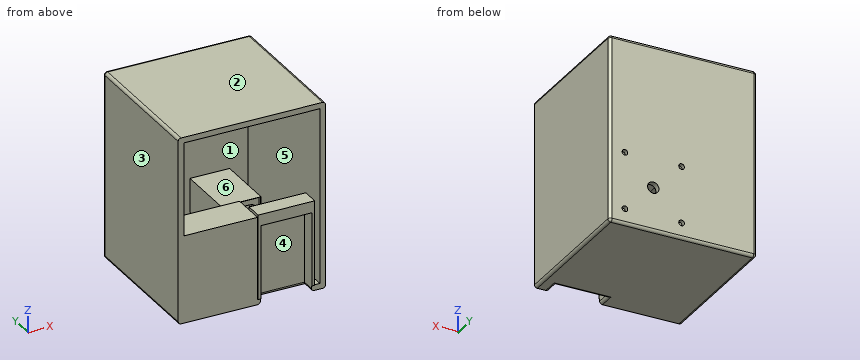
Autodesk Inventor part; units mm, degrees
ref_plane "YZ Plane" through (0, 0, 0) normal (1, 0, 0) x (0, 1, 0)
ref_plane "XZ Plane" through (0, 0, 0) normal (0, 1, 0) x (-1, 0, 0)
ref_plane "XY Plane" through (0, 0, 0) normal (0, 0, 1) x (1, 0, 0)
sketch "Sketch1" plane through (0, 0, 0) normal (0, 1, 0) x (-1, 0, 0)
  line L0 (130, 165) -> (-130, 165)
  line L1 (-130, 165) -> (-130, -165)
  line L2 (-130, -165) -> (130, -165)
  line L3 (130, -165) -> (130, 165)
  point P0 (0, 0)
  point P1 (0, -165)
  point P2 (-130, 0)
  dimension "d0" = 260
  dimension "d1" = 330
extrude "Extrusion1" add sketch "Sketch1" along normal blind 250
sketch "Sketch2" plane through (0, 0, 0) normal (0, -1, 0) x (1, 0, 0)
  line L0 (-120, 155) -> (120, 155)
  line L1 (120, 155) -> (120, -155)
  line L2 (120, -155) -> (-120, -155)
  line L3 (-120, -155) -> (-120, 155)
  line L4 (-130, 165) -> (130, 165)
  line L5 (130, 165) -> (130, -165)
  point P0 (0, 0)
  point P1 (0, 155)
  point P2 (-120, 0)
  dimension "d4" = 10
  dimension "d5" = 10
extrude "Extrusion2" cut sketch "Sketch2" against normal blind 240
fillet "Fillet1" radius 5 8 edges at (0, 250, 165) (-130, 250, 0) (130, 250, 0) (0, 250, -165) (130, 125, -165) (130, 125, 165) (-130, 125, 165) (-130, 125, -165)
sketch "Sketch3" plane through (0, 250, 0) normal (0, 1, 0) x (1, 0, 0)
  circle A0 centre (2.5, 37.5) radius 5
  circle A1 centre (2.5, 137.5) radius 5
  circle A2 centre (102.5, 37.5) radius 5
  circle A3 centre (102.5, 137.5) radius 5
  line L0 (125, 160) -> (125, -160)
  line L1 (-125, 160) -> (125, 160)
  circle A4 centre (52.5, 87.5) radius 10
  point P0 (0, 0)
  dimension "d9" = 10
  dimension "d10" = 10
  dimension "d11" = 10
  dimension "d12" = 10
  dimension "d13" = 100
  dimension "d14" = 100
  dimension "d15" = 22.5
  dimension "d16" = 22.5
  dimension "d19" = 20
  dimension "d20" = 50
  dimension "d21" = 50
extrude "Extrusion3" cut sketch "Sketch3" against normal blind 8
sketch "Sketch4" plane through (52.5, 242, -87.5) normal (0, 1, 0) x (1, 0, 0)
  circle A0 centre (0, 0) radius 10
  circle A1 centre (0, 0) radius 15
  point P0 (-52.5, -87.5)
extrude "Extrusion4" cut sketch "Sketch4" against normal up to next contours A0
sketch "Sketch5" plane through (0, 240, 0) normal (0, -1, 0) x (1, 0, 0)
  line L0 (87.5, -117.5) -> (17.5, -117.5)
  line L1 (17.5, -117.5) -> (17.5, -57.5)
  line L2 (17.5, -57.5) -> (87.5, -57.5)
  line L3 (87.5, -57.5) -> (87.5, -117.5)
  line L4 (120, -155) -> (-120, -155)
  circle A0 centre (52.5, -87.5) radius 15
  circle A1 centre (52.5, -87.5) radius 10
  point P0 (0, 0)
  point P1 (17.5, -87.5)
  point P2 (52.5, -57.5)
  point P3 (52.5, -117.5)
  dimension "d24" = 70
  dimension "d25" = 60
  dimension "d52" = 70
extrude "Extrusion5" add sketch "Sketch5" along normal blind 150 contours L0 L1 L2 L3
sketch "Sketch7" plane through (0, 90, 0) normal (0, -1, 0) x (1, 0, 0)
  line L0 (85, -105) -> (20, -105)
  line L1 (20, -105) -> (20, -70)
  line L2 (20, -70) -> (85, -70)
  line L3 (85, -70) -> (85, -105)
  line L4 (17.5, -117.5) -> (87.5, -117.5)
  line L5 (17.5, -57.5) -> (17.5, -117.5)
  point P0 (0, 0)
  point P1 (52.5, -105)
  point P2 (52.5, -117.5)
  point P3 (52.5, -117.5)
  point P4 (17.5, -87.5)
  point P5 (20, -87.5)
  point P6 (100, -102.5)
  dimension "d28" = 65
  dimension "d29" = 35
extrude "Extrusion6" cut sketch "Sketch7" against normal blind 150
sketch "Sketch8" plane through (0, 240, 0) normal (0, -1, 0) x (1, 0, 0)
  point P0 (0, 0)
sketch "Sketch9" plane through (0, 240, 0) normal (0, -1, 0) x (1, 0, 0)
  circle A0 centre (67, -87.5) radius 2.5
  circle A1 centre (38, -87.5) radius 2.5
  circle A2 centre (52.5, -87.5) radius 10
  circle A3 centre (52.5, -87.5) radius 10
  point P0 (0, 0)
  dimension "d32" = 5
  dimension "d33" = 5
  dimension "d43" = 14.5
  dimension "d44" = 14.5
extrude "Extrusion7" add sketch "Sketch9" along normal up to surface (150 mm away) contours A0 | A1
fillet "Fillet2" radius 15 4 edges at (20, 165, -70) (20, 165, -105) (85, 165, -70) (85, 165, -105)
sketch "Sketch10" plane through (0, 90, 0) normal (0, -1, 0) x (1, 0, 0)
  point P0 (0, 0)
sketch "Sketch11" plane through (0, 90, 0) normal (0, -1, 0) x (1, 0, 0)
  line L0 (18.5, -58.5) -> (86.5, -58.5)
  line L1 (86.5, -58.5) -> (86.5, -116.5)
  line L2 (86.5, -116.5) -> (18.5, -116.5)
  line L3 (18.5, -116.5) -> (18.5, -58.5)
  line L4 (17.5, -57.5) -> (17.5, -117.5)
  line L5 (87.5, -117.5) -> (87.5, -57.5)
  line L6 (87.5, -57.5) -> (17.5, -57.5)
  line L7 (17.5, -117.5) -> (87.5, -117.5)
  point P0 (0, 0)
  point P1 (100, -42.5)
  point P2 (100, -102.5)
  dimension "d46" = 1
  dimension "d47" = 1
  dimension "d48" = 1
  dimension "d49" = 1
extrude "Extrusion8" add sketch "Sketch11" along normal blind 5
sketch "Sketch12" plane through (-120, 0, 155) normal (1, 0, 0) x (0, 0, -1)
  line L0 (315, 0) -> (165, 0)
  line L1 (165, 0) -> (165, 60)
  line L2 (165, 60) -> (315, 60)
  line L3 (315, 60) -> (315, 0)
  line L4 (315, 245) -> (315, 0)
  point P0 (155, 0)
  dimension "d53" = 150
  dimension "d54" = 60
  dimension "d57" = 0
extrude "Extrusion9" add sketch "Sketch12" along normal blind 130
sketch "Sketch15" plane through (0, 85, 0) normal (0, -1, 0) x (1, 0, 0)
  line L0 (97.9773, -47.1324) -> (13.5699, -47.1324)
  line L1 (13.5699, -47.1324) -> (13.5699, -120.1648)
  line L2 (13.5699, -120.1648) -> (97.9773, -120.1648)
  line L3 (97.9773, -120.1648) -> (97.9773, -47.1324)
  point P0 (0, 0)
extrude "Extrusion11" cut sketch "Sketch15" against normal blind 50
sketch "Sketch17" plane through (0, 135, 0) normal (0, -1, 0) x (1, 0, 0)
  line L0 (87.5, -57.5) -> (87.5, -117.5)
  line L1 (87.5, -117.5) -> (17.5, -117.5)
  line L2 (87.5, -57.5) -> (17.5, -57.5)
  line L3 (17.5, -57.5) -> (17.5, -117.5)
  line L4 (17.5, -117.5) -> (87.5, -117.5)
  line L5 (87.5, -117.5) -> (87.5, -57.5)
  line L6 (87, -58) -> (18, -58)
  line L7 (18, -58) -> (18, -117)
  line L8 (18, -117) -> (87, -117)
  line L9 (87, -117) -> (87, -58)
  point P0 (0, 0)
  dimension "d70" = 0.5
  dimension "d71" = 0.5
  dimension "d72" = 0.5
  dimension "d73" = 0.5
extrude "Extrusion12" cut sketch "Sketch17" against normal blind 5 contours L9 L8 L7 L6
chamfer "Chamfer2" distance 0.2 angle 45 4 edges at (52.5, 135, -117) (87, 135, -87.5) (52.5, 135, -58) (18, 135, -87.5)
sketch "Sketch18" plane through (-120, 240, -155) normal (0, 0, 1) x (1, 0, 0)
  line L0 (-10.236, -242) -> (249.4607, -242)
  line L1 (230, -242) -> (130, -242)
  line L2 (130, -242) -> (130, -212)
  line L3 (130, -212) -> (230, -212)
  line L4 (230, -212) -> (230, -242)
  line L5 (250, 5) -> (250, -240)
  line L6 (245, -240) -> (245, 5)
  point P0 (120, -240)
  dimension "d79" = 100
  dimension "d80" = 30
  dimension "d91" = 15
extrude "Extrusion13" add sketch "Sketch18" along normal blind 150
sketch "Sketch19" plane through (125, 245, -165) normal (0, 0, -1) x (-1, 0, 0)
  line L0 (115, -247) -> (15, -247)
  line L1 (115, -217) -> (115, -247)
  line L2 (115, -247) -> (15, -247)
  line L3 (15, -247) -> (15, -217)
  line L4 (15, -217) -> (115, -217)
  line L5 (20, -222) -> (110, -222)
  line L6 (110, -222) -> (110, -265.9747)
  line L7 (110, -265.9747) -> (20, -265.9747)
  line L8 (20, -265.9747) -> (20, -222)
  point P0 (125, -245)
  dimension "d84" = 5
  dimension "d85" = 5
  dimension "d87" = 5
extrude "Extrusion14" cut sketch "Sketch19" against normal blind 140 contours L6 L7 L8 L0 | L0 L8 L5 L6
fillet "Fillet3" radius 5 3 edges at (105, 11.5, -165) (60, 23, -165) (15, 11.5, -165)
properties part number "case" material "Gold"
Can you work these out from the model? Positions are in its coordinate system, mm. Face numbers are marked on the shaded views. A direction names the side the tool comes from. Coordinates: 2 decimals unless noted, no trailing zeros. Write each loop counter-clockwise with the first axis right and the second up, starting at its lowest first coordinate (ties: lowest second). Pieces come first, ordered by that corner, then holes.
Q1. For P1, Ø8, axis at x = 60.5, z = 87.5, coming from the -Y side; P2, Ø6, axis at x = 2.5, z = -37.5, coming from the +Y side, each with a flat end and sliding along its axis, tell me the tip position at first contact or that it passes through.
Results found:
P1: stops at y = 240
P2: stops at y = 242
Q2. If we mould it in two halves opening along X, with no side actions, what happens to the marked faces 1, 2 and 3? For each: +X half, -X half, draft (parallel to the pull), parting line (faces both ways), or undercut.
Results found:
face 1: undercut
face 2: draft
face 3: -X half
Q3. Imagine slicing it at B-B, the plane y = 112. List the corners of the cut face in (x, z) for me.
Results found:
outline: (-130, -160) arc R5 ccw to (-125, -165) - (125, -165) arc R5 ccw to (130, -160) - (130, 160) arc R5 ccw to (125, 165) - (-125, 165) arc R5 ccw to (-130, 160) - close; hole (-120, -155) - (120, -155) - (120, 155) - (-120, 155) - close
Q4. Imagine slicing it at A-A, the plane y = 155.5. List the corners of the cut face in (x, z) for me, plus the area to 3 significant figures.
Results found:
outline: (-130, -160) arc R5 ccw to (-125, -165) - (125, -165) arc R5 ccw to (130, -160) - (130, 160) arc R5 ccw to (125, 165) - (-125, 165) arc R5 ccw to (-130, 160) - close; (17.5, -117.5) - (87.5, -117.5) - (87.5, -57.5) - (17.5, -57.5) - close; circle Ø5 at (38, -87.5); circle Ø5 at (67, -87.5); hole (-120, -155) - (120, -155) - (120, 155) - (-120, 155) - close; hole (20, -90) arc R15 ccw to (35, -105) - (70, -105) arc R15 ccw to (85, -90) - (85, -85) arc R15 ccw to (70, -70) - (35, -70) arc R15 ccw to (20, -85) - close
area: 13,500 mm2
Q5. Please list where these lines run through material, in increasing order: L1, parallel to Z at x = 2.5, y = 244.75; L2, parallel to Z at x = 67, y = 160.5; L3, parallel to Y at x = 99, z = -82.5.
Results found:
L1: z = -165 to -142.5, -132.5 to -42.5, -32.5 to 165
L2: z = -165 to -155, -117.5 to -105, -90 to -85, -70 to -57.5, 155 to 165
L3: y = 23 to 28, 240 to 250
Q6. Which directions (+Z, -Z, +X, -X, +Y, -Y) give clear straight access to the entire face, cutting with the end or side of a thin tool? Please do the marked faces 4, 5 and 6.
Results found:
face 4: -Z, -Y
face 5: -Y
face 6: none
Q7. Imagine slicing it at D-D, the plane z = 121. List the corners of the cut face in (x, y) for me, plus the area to 3 significant figures.
Results found:
outline: (-130, 0) - (-120, 0) - (-120, 240) - (120, 240) - (120, 0) - (130, 0) - (130, 245) arc R5 ccw to (125, 250) - (-125, 250) arc R5 ccw to (-130, 245) - close
area: 7,390 mm2
